Part model, mm, in its own coordinate system. A direction names the side the tool comes from. Give positions to 0.01 mm unless a question says otherwise; leave off trailing zeros. Write each loop counter-clockwise with the first axis right and the second up, starting at its lowest first coordinate (ties: lowest second). Pieces come first, ordered by that corner, then holes.
from build123d import *
from build123d.topology import SkipClean

# Parameters (mm, degrees)
RESSALTO_EXTRUS_O1_START = -10.4
RESSALTO_EXTRUS_O1_DEPTH = 10.4
PADR_OCIRCULAR1_COUNT    = 15
CORTE_EXTRUS_O1_DEPTH    = 22
ESBO_O4_R                = 3.25
CORTE_EXTRUS_O2_DEPTH    = 4
CORTE_EXTRUS_O4_DEPTH    = 20


with BuildPart() as part:
    # Esboço1 → Revolução1 (revolve)
    with BuildSketch(Plane.XY, mode=Mode.PRIVATE) as revolu_o1_sk:
        Polygon((0, 0), (0, 39.4), (5.9, 39.4), (5.9, 33.4), (7.5, 33.4), (7.5, 32.4), (9.374, 32.4), (9.374, 22), (8.47, 22), (8.47, 18.51), (9.9, 18.51), (9.9, 17.01), (8.47, 15.58), (8.47, 0), align=None)
    revolve(revolu_o1_sk.sketch.rotate(Axis((0, 0, 0), (0, 1, 0)), 90), axis=Axis((0, 0, 0), (0, 1, 0)))

    # Esboço2 → Ressalto-extrusão1 (add)
    with BuildSketch(Plane(origin=(0, 32.4, 0), x_dir=(1, 0, 0), z_dir=(0, 1, 0)).offset(RESSALTO_EXTRUS_O1_START)):
        with BuildLine():
            Line((-0.337, 12.746), (0.337, 12.746))
            ThreePointArc((0.337, 12.746), (1.105703178, 11.108702403), (1.167644885, 9.300993572))
            ThreePointArc((1.167644885, 9.300993572), (0, 9.374), (-1.167644885, 9.300993572))
            ThreePointArc((-1.167644885, 9.300993572), (-1.105703178, 11.108702403), (-0.337, 12.746))
        make_face()
    ressalto_extrus_o1 = extrude(amount=RESSALTO_EXTRUS_O1_DEPTH)

    # PadrãoCircular1: Ressalto-extrusão1 ×15 about axis
    padr_ocircular1_axis = Axis((0, 0, 0), (0, 1, 0))
    for i in range(1, PADR_OCIRCULAR1_COUNT):
        add(ressalto_extrus_o1.rotate(padr_ocircular1_axis, i * 360 / PADR_OCIRCULAR1_COUNT))

    # Esboço3 → Corte-extrusão1 (cut)
    with BuildSketch(Plane.XZ):
        with BuildLine():
            Line((2.75, 1.732050808), (2.75, -1.732050808))
            ThreePointArc((2.75, -1.732050808), (-3.25, 0), (2.75, 1.732050808))
        make_face()
    extrude(amount=-CORTE_EXTRUS_O1_DEPTH, mode=Mode.SUBTRACT)

    # Esboço4 → Corte-extrusão2 (cut)
    with SkipClean():  # the faces are left unmerged after this step: merging them gives an invalid solid
        with BuildSketch(Plane.XZ):
            with Locations(Location((0, 0, 0), (0, 0, 270))):
                Circle(ESBO_O4_R)
        extrude(amount=-CORTE_EXTRUS_O2_DEPTH, mode=Mode.SUBTRACT)

    # Esboço7 → Corte-extrusão4 (cut, symmetric)
    with SkipClean():  # the faces are left unmerged after this step: merging them gives an invalid solid
        with BuildSketch(Plane(origin=(0, 0, 0), x_dir=(0, 0, -1), z_dir=(1, 0, 0))):
            with BuildLine():
                Line((-2.1, 5.25), (-2.1, 3.25))
                ThreePointArc((-2.1, 3.25), (0, 1.15), (2.1, 3.25))
                Line((2.1, 3.25), (2.1, 5.25))
                ThreePointArc((2.1, 5.25), (0, 7.35), (-2.1, 5.25))
            make_face()
        extrude(amount=CORTE_EXTRUS_O4_DEPTH, both=True, mode=Mode.SUBTRACT)


solid = part.part
1) 3-axis set-ups, long thin cutter, end or side, ignore diameter. For faces 1 (the cylindrical face through (-0.011, 27.127, 9.374)), 2 (the cylindrical face through (-0.259, 36.358, 5.894)), 3 (the cylindrical face through (-5.44, 7.35, -0.05)): which of +Z, -Z, +X, -X, +Y, -Y reach the whole face in a straight line?
Check result:
face 1: +Z, +Y
face 2: +Y
face 3: +X, -X
2) Mould opens along Y. For faces 4 (the flat face through (8, 32.4, 1)), 5 (the cylindrical face through (-8.11, 27.13, -4.7)), 6 (the flat face through (-5, 4, -2.1)) say: +Y half, -Y half, draft (parallel to the pull), parting line (faces both ways), or undercut.
Check result:
face 4: +Y half
face 5: draft
face 6: undercut
3) Saw through at B-B (y = 35.5). Write the cut outline in (x, z), and give its area (3 significant figures).
Check result:
outline: circle Ø11.8 at (0, 0)
area: 109 mm2
4) Flat gauge pins, fed straight in: P1, Ø2, axis at x = 4.5, y = 20, coming from the -Z side; P2, Ø1, axis at x = -6.5, y = 4.5, coming from the -Z side; P3, Ø1.5, axis at x = -1.5, y = 28.5, coming from the -Z side. Where does each tip first touch, or does it go through?
Check result:
P1: stops at z = -7.71
P2: stops at z = -5.98
P3: stops at z = -12.08
5) Drill centre lines: L1, parallel to X at y = 16.25, z = 0; L2, parallel to X at y = 13.5, z = 0; L3, parallel to Y at x = -9.75, z = 5.75. Where is each one in solid material? Low to high.
Check result:
L1: x = -9.14 to -3.25, 2.75 to 9.14
L2: x = -8.47 to -3.25, 2.75 to 8.47
L3: y = 22 to 32.4
6) Saw through at A-A (y = 12.5). Write the cut outline in (x, z).
Check result:
outline: circle Ø16.94 at (0, 0); hole (2.75, -1.73) - (2.75, 1.73) arc R3.25 ccw (long way) to start
